Could you check a few things on this model? Use its own coordinates, in mm. Round coordinates to 2 decimals unless told otherwise and drop trailing zeros. Write each loop counter-clockwise with the first axis right and the second up, starting at its lowest first coordinate (ties: lowest second). Pieces come first, ordered by that corner, then holes. Notation, with made-up numbers: (-2, 28.5) -> (57, 28.5) arc R25 cw to (57, 59.5) -> close; hole circle Ø11 at (72, 46). An arc over 180 degrees is marked (long way). Answer as CSV lines item,"result". Start each with the question number.
Q1. If I drill on line 1 (X direction, y = 36, z = 358); line 2 (X direction, y = 0.5, z = 441.5); line 3 (Y direction, x = 0, z = -95), over which ranges is the centre line in solid material (lowest first)? Write a range as [from, to].
Q2. Imagine slicing it at A-A on x = 0. Please give me the cut outline in (y, z), and give its area (3 significant figures).
Q3. Will these pins go through, and if not, where does the flat tip stop? pin 1 Ø2 at (x, z) = (-14, -60) entering from +Y; pin 2 Ø2.5 at (y, z) = (-15.5, -19.5) entering from -X; pin 3 Ø7.5 at (y, z) = (-2, 73.5) entering from +X; pin 4 Ø1.1 at (y, z) = (44, 178) entering from -X.
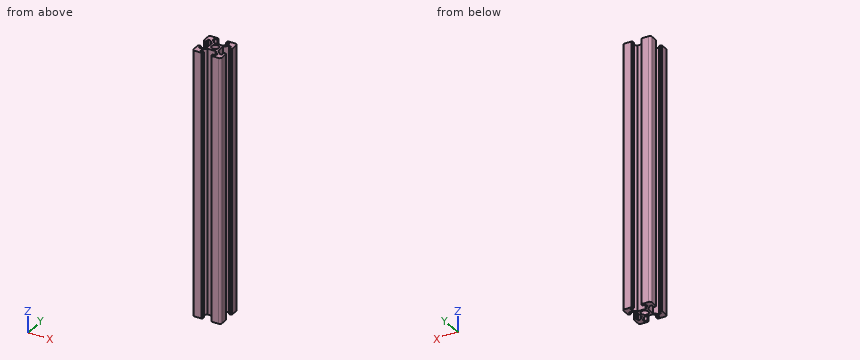
from build123d import *

# Parameters (mm, degrees)
SKETCH1_R           = 2.5
BOSS_EXTRUDE1_DEPTH = 189.096108091
SCALE_2_SCALE       = 3
SCALE_3_SCALE       = 6
SCALE_5_SCALE       = 2
SCALE_6_SCALE       = 0.25
SCALE_7_SCALE       = 0.125
SCALE_8_SCALE       = 0.25
SCALE_9_SCALE       = 4
SCALE_10_SCALE      = 4


with BuildPart() as part:
    # Sketch1 → Boss-Extrude1 (new body)
    with BuildSketch(Plane.XY):
        with BuildLine():
            Line((2.839339828, 3.9), (5.5, 6.560660172))
            Line((5.5, 6.560660172), (5.5, 8.2))
            Line((5.5, 8.2), (3.1, 8.2))
            Line((3.1, 8.2), (3.1, 9.5))
            Line((3.1, 9.5), (3.6, 9.5))
            Line((3.6, 9.5), (3.6, 10))
            Line((3.6, 10), (8.5, 10))
            ThreePointArc((8.5, 10), (9.560660172, 9.560660172), (10, 8.5))
            Line((10, 8.5), (10, 3.6))
            Line((10, 3.6), (9.5, 3.6))
            Line((9.5, 3.6), (9.5, 3.1))
            Line((9.5, 3.1), (8.2, 3.1))
            Line((8.2, 3.1), (8.2, 5.5))
            Line((8.2, 5.5), (6.560660172, 5.5))
            Line((6.560660172, 5.5), (3.9, 2.839339828))
            Line((3.9, 2.839339828), (3.9, -2.839339828))
            Line((3.9, -2.839339828), (6.560660172, -5.5))
            Line((6.560660172, -5.5), (8.2, -5.5))
            Line((8.2, -5.5), (8.2, -3.1))
            Line((8.2, -3.1), (9.5, -3.1))
            Line((9.5, -3.1), (9.5, -3.6))
            Line((9.5, -3.6), (10, -3.6))
            Line((10, -3.6), (10, -8.5))
            ThreePointArc((10, -8.5), (9.560660172, -9.560660172), (8.5, -10))
            Line((8.5, -10), (3.6, -10))
            Line((3.6, -10), (3.6, -9.5))
            Line((3.6, -9.5), (3.1, -9.5))
            Line((3.1, -9.5), (3.1, -8.2))
            Line((3.1, -8.2), (5.5, -8.2))
            Line((5.5, -8.2), (5.5, -6.560660172))
            Line((5.5, -6.560660172), (2.839339828, -3.9))
            Line((2.839339828, -3.9), (-2.839339828, -3.9))
            Line((-2.839339828, -3.9), (-5.5, -6.560660172))
            Line((-5.5, -6.560660172), (-5.5, -8.2))
            Line((-5.5, -8.2), (-3.1, -8.2))
            Line((-3.1, -8.2), (-3.1, -9.5))
            Line((-3.1, -9.5), (-3.6, -9.5))
            Line((-3.6, -9.5), (-3.6, -10))
            Line((-3.6, -10), (-8.5, -10))
            ThreePointArc((-8.5, -10), (-9.560660172, -9.560660172), (-10, -8.5))
            Line((-10, -8.5), (-10, -3.6))
            Line((-10, -3.6), (-9.5, -3.6))
            Line((-9.5, -3.6), (-9.5, -3.1))
            Line((-9.5, -3.1), (-8.2, -3.1))
            Line((-8.2, -3.1), (-8.2, -5.5))
            Line((-8.2, -5.5), (-6.560660172, -5.5))
            Line((-6.560660172, -5.5), (-3.9, -2.839339828))
            Line((-3.9, -2.839339828), (-3.9, 2.839339828))
            Line((-3.9, 2.839339828), (-6.560660172, 5.5))
            Line((-6.560660172, 5.5), (-8.2, 5.5))
            Line((-8.2, 5.5), (-8.2, 3.1))
            Line((-8.2, 3.1), (-9.5, 3.1))
            Line((-9.5, 3.1), (-9.5, 3.6))
            Line((-9.5, 3.6), (-10, 3.6))
            Line((-10, 3.6), (-10, 8.5))
            ThreePointArc((-10, 8.5), (-9.560660172, 9.560660172), (-8.5, 10))
            Line((-8.5, 10), (-3.6, 10))
            Line((-3.6, 10), (-3.6, 9.5))
            Line((-3.6, 9.5), (-3.1, 9.5))
            Line((-3.1, 9.5), (-3.1, 8.2))
            Line((-3.1, 8.2), (-5.5, 8.2))
            Line((-5.5, 8.2), (-5.5, 6.560660172))
            Line((-5.5, 6.560660172), (-2.839339828, 3.9))
            Line((-2.839339828, 3.9), (2.839339828, 3.9))
        make_face()
        with Locations((0, 0.235847297)):
            Circle(SKETCH1_R, mode=Mode.SUBTRACT)
    extrude(amount=BOSS_EXTRUDE1_DEPTH)


with BuildPart() as part_1:
    # 缩放比例2: scaled about (0, -0.027095247, 94.548054046)
    add(part.part.scale(SCALE_2_SCALE).moved(Location((0, 0.054190494, -189.096108092))))


with BuildPart() as part_2:
    # 缩放比例3: scaled about (0, -0.027095247, 94.548054045)
    add(part_1.part.scale(SCALE_3_SCALE).moved(Location((0, 0.135476235, -472.740270225))))


with BuildPart() as part_3:
    # 缩放比例5: scaled about (0, -0.027095249, 94.548054043)
    add(part_2.part.scale(SCALE_5_SCALE).moved(Location((0, 0.027095249, -94.548054043))))


with BuildPart() as part_4:
    # 缩放比例6: scaled about (0, -0.027095249, 94.548054044)
    add(part_3.part.scale(SCALE_6_SCALE).moved(Location((0, -0.020321437, 70.911040533))))


with BuildPart() as part_5:
    # 缩放比例7: scaled about (0, -0.027095249, 94.548054044)
    add(part_4.part.scale(SCALE_7_SCALE).moved(Location((0, -0.023708343, 82.729547289))))


with BuildPart() as part_6:
    # 缩放比例8: scaled about (0, -0.027095249, 94.548054044)
    add(part_5.part.scale(SCALE_8_SCALE).moved(Location((0, -0.020321437, 70.911040533))))


with BuildPart() as part_7:
    # 缩放比例9: scaled about (0, -0.027095249, 94.548054044)
    add(part_6.part.scale(SCALE_9_SCALE).moved(Location((0, 0.081285747, -283.644162132))))


with BuildPart() as part_8:
    # 缩放比例10: scaled about (0, -0.027095249, 94.548054044)
    add(part_7.part.scale(SCALE_10_SCALE).moved(Location((0, 0.081285747, -283.644162132))))


solid = part_8.part
Checks:
1,line 1,"[-45, -24.75], [24.75, 45]"
1,line 2,"[-17.55, -11.23], [11.23, 17.55]"
1,line 3,"[-17.46, -10.09], [12.41, 17.64]"
2,outline,"(-17.46, -330.92) -> (-10.09, -330.92) -> (-10.09, 520.01) -> (-17.46, 520.01) -> close; (12.41, -330.92) -> (17.64, -330.92) -> (17.64, 520.01) -> (12.41, 520.01) -> close"
2,area,"10,700 mm^2"
3,pin 1,"y = 42.84"
3,pin 2,"x = -45"
3,pin 3,"x = 17.55"
3,pin 4,"x = -42.67"
